Can you work these out from the model? Positions are in its coordinate system, mm. A direction names the side the tool comes from. Round coordinates to 2 decimals unless told otherwise and drop trailing zeros. Loops run counter-clockwise (first coordinate to the right, second up) from the corner with the lowest first, then second, coordinate; pieces in that order, holes last.
(1) I want a section at A-A on x = 0. Write out the boundary of the cut face in (y, z).
(2) Which directions (+Z, -Z, +X, -X, +Y, -Y) give clear straight access to the entire face, cutting with the end or side of a thin tool? Please do faces 4 (the face through (-1.08, 43.21, -4.88)), 5 (the face through (9, 14.5, 0)), 6 (the face through (-0.188, 29.645, -4.896)), 7 (the face through (-2.75, 20, 8)), 8 (the face through (0.489, -22.245, -0.133)).
(3) If I drill on line 1 along Y through (x, z) = (0, 3.75); line 2 along Z through (x, y) = (0, 54.35); line 3 along Y through (x, z) = (0, 5.25), over which ranges is the centre line in solid material (lowest first)?
(4) Will these pins go through, and if not, where does the flat tip stop? pin 1 Ø3 at (x, y) = (17.75, 0) entering from +Z; pin 2 Ø4 at (x, z) = (-3, -5) entering from -Y; pin 3 Ø0.6 at (y, z) = (21, 8.5) entering from +X; pin 4 Ø7 at (x, z) = (0, 0) entering from +Y.
(5) I want a section at C-C on y = -12.5. Write out the boundary of the cut face in (x, z), plus the area to 3 significant figures.
(6) Thinking about a two-plate mould opening in X: for faces 1 (the face through (-22.25, 5, 0)), 2 (the face through (-10, 12, 0)), 3 (the face through (3, 46.25, 3)), which applies, released by +X, released by -X, zero draft, split by the parting line, or undercut?
(7) I want a section at D-D on z = 0. Give the number of separate pieces and of enclosed holes in the cut face, plus the area to 3 significant figures.
(8) I want a section at B-B on y = 7.5. Write out the boundary of the cut face in (x, z).
Autodesk Inventor part; units mm, degrees
ref_plane "YZ Plane" through (0, 0, 0) normal (1, 0, 0) x (0, 1, 0)
ref_plane "XZ Plane" through (0, 0, 0) normal (0, 1, 0) x (-1, 0, 0)
ref_plane "XY Plane" through (0, 0, 0) normal (0, 0, 1) x (1, 0, 0)
sketch "Skizze1" plane through (0, 0, 0) normal (0, 0, 1) x (1, 0, 0)
  circle A0 centre (17.75, 0) radius 1.75
  circle A1 centre (-17.75, 0) radius 1.75
  circle A2 centre (0, 0) radius 14.25
  arc A3 (-22.25, 0) -> (22.25, 0) centre (0, 0) ccw
  line L0 (-22.25, 25.25) -> (22.25, 25.25)
  line L1 (22.25, 25.25) -> (22.25, 22.25)
  line L2 (22.25, 22.25) -> (-22.25, 22.25)
  line L3 (-22.25, 22.25) -> (-22.25, 25.25)
  line L4 (0, -31.75) -> (0, 34.75)
  line L5 (-22.25, 22.25) -> (-22.25, 0)
  line L6 (22.25, 22.25) -> (22.25, 0)
  dimension "d2" = 3.5
  dimension "d3" = 3.5
  dimension "d8" = 28.5
  dimension "d9" = 44.5
  dimension "d10" = 44.5
  dimension "d11" = 3
extrude "Extrusion2" add sketch "Skizze1" along normal mid plane 19 contours A2 L4 L2 L6 A3 | A2 L4 A3 L5 L2
sketch "Skizze2" plane through (0, 0, 9.5) normal (0, 0, 1) x (1, 0, 0)
  line L0 (-8.5, 18.4) -> (8.5, 18.4)
  line L1 (8.5, 18.4) -> (8.5, 11.4)
  line L2 (8.5, 11.4) -> (-8.5, 11.4)
  line L3 (0, -31.15) -> (0, 31.15)
  line L4 (-31.15, 0) -> (31.15, 0)
  line L5 (-10, 14.5) -> (-8.5, 14.5)
  line L6 (-10, 14.5) -> (-10, 10)
  line L7 (-10, 10) -> (-8.5, 10)
  line L8 (-8.5, 18.4) -> (-8.5, 11.4)
  line L9 (-8.5, 14.5) -> (-8.5, 10)
  line L10 (10, 14.5) -> (8.5, 14.5)
  line L11 (10, 14.5) -> (10, 10)
  line L12 (10, 10) -> (8.5, 10)
  line L13 (8.5, 14.5) -> (8.5, 10)
  point P0 (0, 0)
  point P1 (0, 11.4)
  point P2 (0, 18.4)
  dimension "d14" = 17
  dimension "d15" = 7
  dimension "d16" = 11.4
  dimension "d34" = 1.5
  dimension "d45" = 4.5
  dimension "d46" = 10
  dimension "d48" = 1.5
extrude "Extrusion3" cut sketch "Skizze2" against normal blind 19
sketch "Skizze3" plane through (-8.5, 18.4, 9.5) normal (0, -1, 0) x (1, 0, 0)
  line L0 (0, 0) -> (17, 0)
  line L1 (5.75, 0) -> (11.25, 0)
  line L2 (11.25, 0) -> (11.25, -3)
  line L3 (11.25, -3) -> (5.75, -3)
  line L4 (5.75, -3) -> (5.75, 0)
  line L5 (0, 0) -> (0, -19)
  point P0 (8.5, -9.5)
  dimension "d19" = 5.5
  dimension "d20" = 3
  dimension "d38" = 5.75
extrude "Extrusion4" cut sketch "Skizze3" against normal blind 4
fillet "Rundung1" radius 2 2 edges at (-8.5, 18.4, 0) (8.5, 18.4, 0)
sketch "Skizze4" plane through (-22.25, 22.25, -9.5) normal (0, 1, 0) x (1, 0, 0)
  line L0 (0, -19) -> (0, 0)
  line L1 (0, 0) -> (44.5, 0)
  line L2 (44.5, -19) -> (0, -19)
  line L3 (44.5, 0) -> (44.5, -19)
  circle A0 centre (22.25, -9.5) radius 4.9
  point P0 (25, -19)
  dimension "d39" = 9.8
fillet "Rundung2" radius 1 2 edges at (-2.75, 20.325, 6.5) (2.75, 20.325, 6.5)
extrude "Extrusion7" add sketch "Skizze4" along normal blind 15 contours A0
sketch "Skizze5" plane through (0, 37.25, 0) normal (0, 1, 0) x (1, 0, 0)
  circle A0 centre (0, 0) radius 6.5
  dimension "d51" = 13
extrude "Extrusion8" add sketch "Skizze5" along normal blind 3
sketch "Skizze6" plane through (0, 40.25, 0) normal (0, 1, 0) x (1, 0, 0)
  circle A0 centre (0, 0) radius 5
  dimension "d54" = 10
extrude "Extrusion9" add sketch "Skizze6" along normal blind 6
sketch "Skizze8" plane through (0, 40.25, 0) normal (0, 1, 0) x (1, 0, 0)
  line L0 (-6.5, 9.5) -> (-6.5, -9.5)
  line L1 (6.5, -9.5) -> (6.5, 9.5)
  line L2 (-6.5, 0) -> (6.5, 0)
  line L3 (6.5, 0) -> (6.5, -6.5)
  line L4 (6.5, -6.5) -> (-6.5, -6.5)
  line L5 (-6.5, -6.5) -> (-6.5, 0)
  line L6 (-6.5, -6.5) -> (6.5, -6.5)
  line L7 (6.5, -6.5) -> (6.5, -4.5)
  line L8 (6.5, -4.5) -> (-6.5, -4.5)
  line L9 (-6.5, -4.5) -> (-6.5, -6.5)
  point P0 (0, 0)
  point P1 (-6.5, -4.5)
  point P2 (-6.5, -6.5)
  dimension "d60" = 6.5
  dimension "d61" = 2
sketch "Skizze9" plane through (0, 46.25, 0) normal (0, 1, 0) x (1, 0, 0)
  circle A0 centre (0, 0) radius 3.9
  dimension "d62" = 7.8
extrude "Extrusion11" add sketch "Skizze9" along normal blind 11
sketch "Skizze10" plane through (0, 57.25, 0) normal (0, 1, 0) x (1, 0, 0)
  circle A0 centre (0, 0) radius 2.25
  dimension "d65" = 4.5
extrude "Extrusion12" cut sketch "Skizze10" against normal blind 6
extrude "Extrusion13" cut sketch "Skizze8" against normal blind 18 contours L8 L1 L4 L0
fillet "Rundung6" radius 13 2 edges at (-22.25, 22.25, 0) (22.25, 22.25, 0)
properties part number "_3D-Druck"
Filled sheet:
1. outline: (-22.25, -9.5) - (-14.25, -9.5) - (-14.25, 9.5) - (-22.25, 9.5) - close; (18.4, -9.5) - (22.25, -9.5) - (22.25, -4.9) - (37.25, -4.9) - (37.25, -6.5) - (40.25, -6.5) - (40.25, -5) - (46.25, -5) - (46.25, -3.9) - (57.25, -3.9) - (57.25, -2.25) - (51.25, -2.25) - (51.25, 2.25) - (57.25, 2.25) - (57.25, 3.9) - (46.25, 3.9) - (46.25, 5) - (40.25, 5) - (40.25, 4.5) - (22.25, 4.5) - (22.25, 6.5) - (18.4, 6.5) - close
2. face 4: +Y
2. face 5: +Z, -Z
2. face 6: none
2. face 7: +Z, +Y
2. face 8: +Z, -Z, -Y
3. line 1: y = -22.25 to -14.25, 18.4 to 57.25
3. line 2: z = -3.9 to -2.25, 2.25 to 3.9
3. line 3: y = -22.25 to -14.25, 18.4 to 22.25
4. pin 1: passes through
4. pin 2: stops at y = -22.23
4. pin 3: stops at x = 15.41
4. pin 4: stops at y = 57.25
5. outline: (-18.41, -9.5) - (-6.84, -9.5) - (-6.84, 9.5) - (-18.41, 9.5) - close; (6.84, -9.5) - (18.41, -9.5) - (18.41, 9.5) - (6.84, 9.5) - close
5. area: 439 mm2
6. face 1: released by -X
6. face 2: undercut
6. face 3: zero draft
7. separate pieces: 1
7. enclosed holes: 3
7. area: 1,250 mm2
8. outline: (-22.25, -9.5) - (-12.12, -9.5) - (-12.12, 9.5) - (-22.25, 9.5) - close; (12.12, -9.5) - (22.25, -9.5) - (22.25, 9.5) - (12.12, 9.5) - close
